For this review, use the dimensioned drawing (mm, ordinates from the lowest corner) and the shaded views. Round coordinates to 2 decimals unless told otherwise and drop trailing zeros. Loops run counter-clockwise (first coordinate to the right, second up) from the corner with the lowest first, then second, coordinate; pieces in that order, holes last. Notation, with made-up numbers: (13.5, -6) - (63.5, -6) arc R22 cw to (63.5, 12) - close; hole circle Ø9 at (-8, 76.5). An arc over 180 degrees is marked (long way). Use one line per item in the form item = value. Start each with the question number.
(1) The part is to be moulded in two halves that separate along Z. For the marked faces 1, 2 and 3, say which applies: released by +Z, released by -Z, zero draft, split by the parting line, or undercut.
(2) We need section A-A, the plane z = 49. Write out the cut boundary in (x, y).
(3) Wall thickness on probe 1 along X at (y, z) = (13.25, 49); probe 2 along Z at (x, y) = (32, 4.5) (1 decimal); probe 3 along Y at (x, z) = (77, 76.5): over which ranges is each line inside the solid? List them lowest first. Write a range as [from, to].
(4) We need section C-C, the plane z = 98.5. Write out the cut boundary in (x, y), then the cut area to 3 significant figures.
(5) For pin 1 (3.5 mm diameter, centred on x = 76, z = 92, fed in from +Y); pin 2 (22.5 mm diameter, centred on x = 38.5, z = 103.5, fed in from +Y), all flat-tipped, find the tip position at first contact; note any pin that passes through.
(6) We need section B-B, the plane x = 59.5. Write out the cut boundary in (y, z).
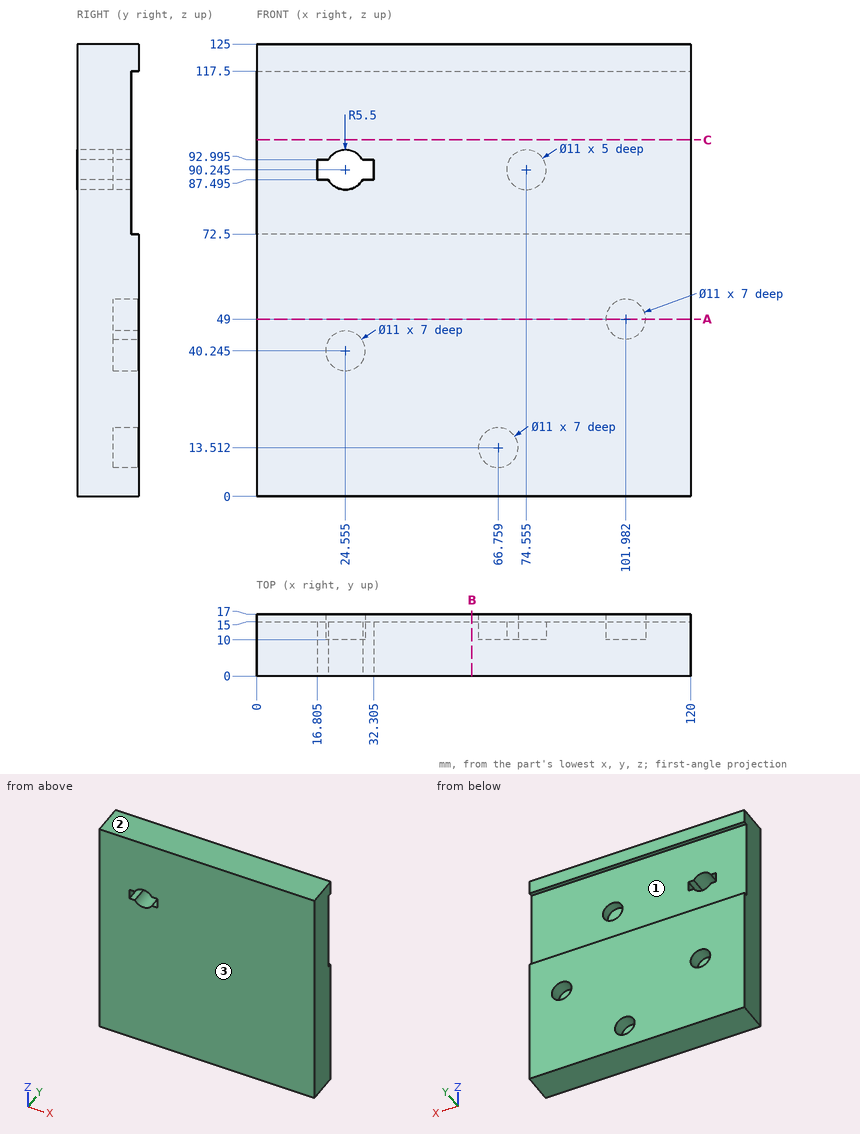
Data:
q1.face_1 = undercut
q1.face_2 = released by +Z
q1.face_3 = zero draft
q2.outline = (0, 0) - (120, 0) - (120, 17) - (107.48, 17) - (107.48, 10) - (96.48, 10) - (96.48, 17) - (0, 17) - close
q3.probe_1 = [0, 96.48], [107.48, 120]
q3.probe_2 = [0, 87.5], [93, 125]
q3.probe_3 = [0, 15]
q4.outline = (0, 0) - (120, 0) - (120, 15) - (0, 15) - close
q4.area = 1,800 mm^2
q5.pin_1 = 10
q5.pin_2 = 15
q6.outline = (0, 0) - (17, 0) - (17, 72.5) - (15, 72.5) - (15, 117.5) - (17, 117.5) - (17, 125) - (0, 125) - close
